```python
from build123d import *

# Parameters (mm, degrees)
F0_R     = 2.5
F1_DEPTH = 14
F3_DEPTH = 25


with BuildPart() as f1:
    # F0 (on Top) → F1 (new body)
    with BuildSketch(Plane.XY):
        Polygon((-11.25, 5), (-23.25, 5), (-23.25, -5), (23.25, -5), (23.25, 5), (11.25, 5), (11.25, -3.5), (-11.25, -3.5), align=None)
        with Locations((-15.75, 0)):
            Circle(F0_R, mode=Mode.SUBTRACT)
        with Locations((15.75, 0)):
            Circle(F0_R, mode=Mode.SUBTRACT)
    extrude(amount=F1_DEPTH)

    # F2 (on face) → F3 (cut)
    with BuildSketch(Plane.XZ.offset(5)):
        with BuildLine():
            Line((-8.5, 14), (-8.5, 12))
            ThreePointArc((-8.5, 12), (0, 3.5), (8.5, 12))
            Line((8.5, 12), (8.5, 14))
            Line((8.5, 14), (-8.5, 14))
        make_face()
    extrude(amount=-F3_DEPTH, mode=Mode.SUBTRACT)


solid = f1.part
```
Model file for the job. Use its own axes, mm. A direction names the side the tool comes from. Coordinates: 2 decimals unless noted, no trailing zeros. Order: outer loops, then holes, each group sorted by start corner. A loop starts at its lowest first (then second) coordinate and runs counter-clockwise, first axis right, second up. Notation, with made-up numbers: (36.25, -18.75) -> (82.25, -18.75) arc R12 cw to (82.25, -11.75) -> close; hole circle Ø11 at (20.25, -1). An arc over 180 degrees is marked (long way). Return JSON: item names as keys, results as strings.
Item 1: Wall check: line 1 along X through (y, z) = (-3, 0.5); line 2 along X through (y, z) = (2, 1.5); line 3 along X through (y, z) = (-1.5, 10.25). Give the ranges that are in metal, low to high. Write a range as from..to.
Model answer:
{"line 1": "x = -23.25..-11.25, 11.25..23.25", "line 2": "x = -23.25..-17.25, -14.25..-11.25, 11.25..14.25, 17.25..23.25", "line 3": "x = -23.25..-17.75, -13.75..-11.25, 11.25..13.75, 17.75..23.25"}
Item 2: Slice it at C-C (y = 4). Write the cut outline in (x, z).
Model answer:
{"outline": "(-23.25, 0) -> (-11.25, 0) -> (-11.25, 14) -> (-23.25, 14) -> close; (11.25, 0) -> (23.25, 0) -> (23.25, 14) -> (11.25, 14) -> close"}
Item 3: Slice it at B-B (z = 8). Write the cut outline in (x, y), then the cut area to 3 significant figures.
Model answer:
{"outline": "(-23.25, -5) -> (-7.5, -5) -> (-7.5, -3.5) -> (-11.25, -3.5) -> (-11.25, 5) -> (-23.25, 5) -> close; (7.5, -5) -> (23.25, -5) -> (23.25, 5) -> (11.25, 5) -> (11.25, -3.5) -> (7.5, -3.5) -> close; hole circle Ø5 at (-15.75, 0); hole circle Ø5 at (15.75, 0)", "area": "212 mm²"}
Item 4: Slice it at A-A (y = 0). Write the cut outline in (x, z).
Model answer:
{"outline": "(-23.25, 0) -> (-18.25, 0) -> (-18.25, 14) -> (-23.25, 14) -> close; (-13.25, 0) -> (-11.25, 0) -> (-11.25, 14) -> (-13.25, 14) -> close; (11.25, 0) -> (13.25, 0) -> (13.25, 14) -> (11.25, 14) -> close; (18.25, 0) -> (23.25, 0) -> (23.25, 14) -> (18.25, 14) -> close"}
Item 5: Mould opens along X. For faces 1 (the face through (23.25, 0, 7)), 2 (the face through (-11.25, 1, 7)), 3 (the face through (19, 0, 14)) say: pulls with the +X half, pulls with the -X half, needs draft (parallel to the pull), parting line crosses it, or undercut.
Model answer:
{"face 1": "pulls with the +X half", "face 2": "undercut", "face 3": "needs draft"}
Item 6: Slice it at D-D (x = -15.75). Write the cut outline in (y, z), then the cut area to 3 significant figures.
Model answer:
{"outline": "(-5, 0) -> (-2.5, 0) -> (-2.5, 14) -> (-5, 14) -> close; (2.5, 0) -> (5, 0) -> (5, 14) -> (2.5, 14) -> close", "area": "70.0 mm²"}
Item 7: 3-axis set-ups, long thin cutter, end or side, ignore diameter. For faces 4 (the face through (8.5, -4, 13)), 5 (the face through (-18.248, 0.11, 6.902)), 6 (the face through (0, -3.5, 2)): which of +Z, -Z, +X, -X, +Y, -Y reach the whole face in a straight line?
Model answer:
{"face 4": "+Z, +Y, -Y", "face 5": "+Z, -Z", "face 6": "+Z, -Z, +Y"}
